Job drawing, mm, ordinate dimensions from the low corner. One solid piece. Round coordinates to 2 decimals unless told otherwise and drop trailing zeros. Order: outer loops, then holes, each group sorted by start corner. A loop starts at its lowest first (then second) coordinate and runs counter-clockwise, first axis right, second up. Notation, with made-up numbers: (54.25, 20) -> (59.25, 20) arc R24 cw to (59.25, 31) -> close; hole circle Ø1 at (80.25, 45). An arc over 180 degrees is marked (long way). Return JSON: item names as keys, results as strings. Group by question number.
Q1. Flat gauge pins, fed straight in: pin 1 (1 mm diameter, centred on x = 9.5, z = 4, fed in from -Y); pin 2 (1.5 mm diameter, centred on y = 16.5, z = 3, fed in from +X); pin 3 (1 mm diameter, centred on x = 13, z = 4.5, fed in from -Y). Where does each tip first touch, or does it go through?
Q2. Probe line 1 along X through (y, z) = (9.25, 1.75); line 2 along X through (y, z) = (5.75, 6.5) (1 decimal); line 3 along Y through (x, z) = (9.25, 6.5) (1 decimal). List the from-to ranges inside material, lowest first.
Q3. Cut at A-A (z = 5). Write the cut outline in (x, y) (1 decimal).
Q4. Mould opens along Y. For the marked faces 1, 2 and 3 say: +Y half, -Y half, draft (parallel to the pull), parting line (faces both ways), or undercut.
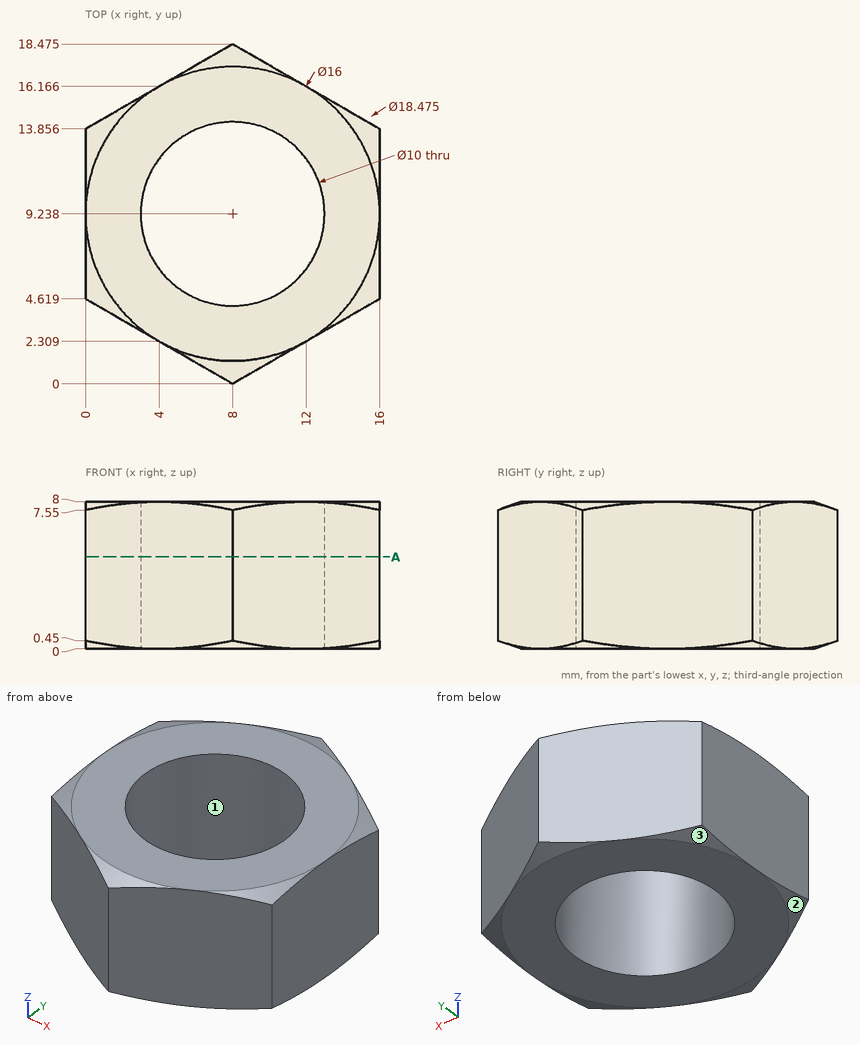
Solution:
{
 "1": {"pin 1": "stops at y = 0.58", "pin 2": "stops at x = 12.72", "pin 3": "stops at y = 2.6"},
 "2": {"line 1": "x = 0 to 3, 13 to 16", "line 2": "x = 0 to 4.4, 11.6 to 16", "line 3": "y = 0.7 to 4.4, 14.1 to 17.8"},
 "3": {"outline": "(0, 4.6) -> (8, 0) -> (16, 4.6) -> (16, 13.9) -> (8, 18.5) -> (0, 13.9) -> close; hole circle Ø10 at (8, 9.2)"},
 "4": {"face 1": "undercut", "face 2": "-Y half", "face 3": "+Y half"}
}
